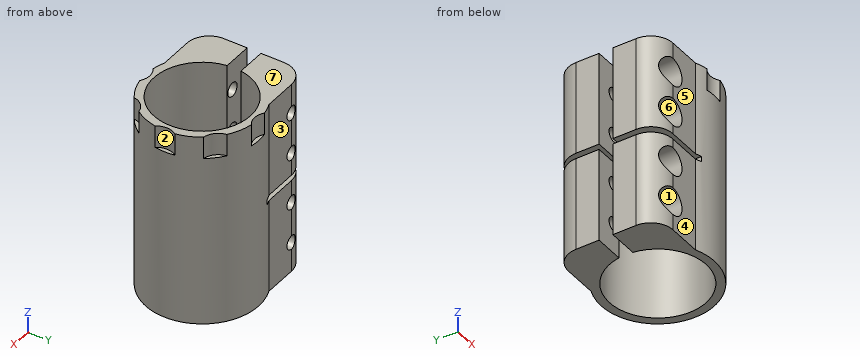
from build123d import *

# Parameters (mm, degrees)
F1_DEPTH       = 35
F3_D           = 5
F3_START       = 1.8205079
F3_CBORE_D     = 10
F3_CBORE_DEPTH = 8
F4_W           = 22.4
F4_H           = 2
F5_DEPTH       = 25
F6_R           = 6
F7_DEPTH       = 8


with BuildPart() as f1:
    # F0 (on Top) → F1 (new body, symmetric)
    with BuildSketch(Plane.XY):
        with BuildLine():
            Line((-20.1192642082, -18.9086026559), (-7.9192642082, -18.9086026559))
            ThreePointArc((-7.9192642082, -18.9086026559), (20.5, 0), (-7.9192642082, 18.9086026559))
            Line((-7.9192642082, 18.9086026559), (-20.1192642082, 18.9086026559))
            ThreePointArc((-20.1192642082, 18.9086026559), (-25.7761184577, 16.5654569054), (-28.1192642082, 10.9086026559))
            Line((-28.1192642082, 10.9086026559), (-28.1192642082, 2.5086026559))
            Line((-28.1192642082, 2.5086026559), (-17.3192642082, 2.5086026559))
            ThreePointArc((-17.3192642082, 2.5086026559), (17.5, 0), (-17.3192642082, -2.5086026559))
            Line((-17.3192642082, -2.5086026559), (-28.1192642082, -2.5086026559))
            Line((-28.1192642082, -2.5086026559), (-28.1192642082, -10.9086026559))
            ThreePointArc((-28.1192642082, -10.9086026559), (-25.7761184577, -16.5654569054), (-20.1192642082, -18.9086026559))
        make_face()
    extrude(amount=F1_DEPTH, both=True)

    # F3 (through all)
    # its depths count from where the whole tool has entered the part; down to there all is cleared
    with Locations(Plane.XZ.offset(18.9086026559).offset(-F3_START)):
        with Locations((-20.2, -24.25), (-20.2, -9.25), (-20.2, 9.25), (-20.2, 24.25)):
            CounterBoreHole(F3_D / 2, F3_CBORE_D / 2, F3_CBORE_DEPTH)

    # F4 (on Front) → F5 (cut, symmetric)
    with BuildSketch(Plane.XZ):
        with Locations((-16.9192642082, 0)):
            Rectangle(F4_W, F4_H)
    extrude(amount=F5_DEPTH, both=True, mode=Mode.SUBTRACT)

    # F6 (on face) → F7 (cut)
    with BuildSketch(Plane.XY.offset(35)):
        with Locations((0, -25)):
            Circle(F6_R)
        with Locations((17.6776695297, -17.6776695297)):
            Circle(F6_R)
        with Locations((25, 0)):
            Circle(F6_R)
        with Locations((17.6776695297, 17.6776695297)):
            Circle(F6_R)
        with Locations((0, 25)):
            Circle(F6_R)
    extrude(amount=-F7_DEPTH, mode=Mode.SUBTRACT)


solid = f1.part
Verification items for the finished model (mm, model axes). Face numbers are marked on the shaded views. A direction names the side the tool comes from. Coordinates: 2 decimals unless noted, no trailing zeros. Write each loop counter-clockwise with the first axis right and the second up, starting at its lowest first coordinate (ties: lowest second). Pieces come first, ordered by that corner, then holes. Notation, with made-up numbers: (11.5, -37) -> (51.5, -37) arc R26 ccw to (51.5, -18) -> close; hole circle Ø3 at (61.25, 39). An arc over 180 degrees is marked (long way). One line per item, written item: value. Start each with the question number.
Q1. Mould release check, pull along Z, two halves, no side actions. Record for the marked faces 5, 6 and 7: pulls with the +Z half, pulls with the -Z half, needs draft (parallel to the pull), parting line crosses it, or undercut.
Q2. Cross-section at D-D on z = 25.5. Enter the section's corners in (x, y).
Q3. Cross-section at C-C on x = 8.5. Enter the section's corners in (y, z), and give its area (3 significant figures).
Q4. Thickness scan on L1, parallel to Z at x = -20.2, y = -16.75; L2, parallel to Z at x = -20, y = -5; L3, parallel to X at y = 14.75, z = -9.25. Record the ranges inside material, lowest first. Write a range as from..to.
Q5. Cross-section at B-B on z = -16. Enter the section's corners in (x, y).
Q6. Go/stop test with flat-tipped pins: P1, Ø3, axis at x = 4, z = 12, coming from the +Y side; P2, Ø5.5, axis at x = -20.5, z = -15, coming from the +Y side; P3, Ø1.6, axis at y = 19, z = 0, coming from the -X side. Record where each tip stops, or that it passes through.
Q7. Access from +Z, -Z, +X, -X, +Y, -Y to the whole of each face (thin tool, end or side, straight path). Record for the marked faces 1, 2, 3 and 4.
Q8. Cross-section at A-A on y = 14. Enter the section's corners in (x, z).
Checked values:
1. face 5: needs draft
1. face 6: undercut
1. face 7: pulls with the +Z half
2. outline: (-28.12, -10.91) arc R8 ccw to (-25.04, -17.22) -> (-25.04, -9.09) -> (-22.37, -9.09) -> (-22.37, -2.51) -> (-28.12, -2.51) -> close; (-28.12, 2.51) -> (-22.37, 2.51) -> (-22.37, 18.59) arc R8 ccw to (-28.12, 10.91) -> close; (-18.03, -9.09) -> (-15.36, -9.09) -> (-15.36, -18.91) -> (-7.92, -18.91) arc R20.5 ccw (long way) to (-7.92, 18.91) -> (-18.03, 18.91) -> (-18.03, 2.51) -> (-17.32, 2.51) arc R17.5 cw (long way) to (-17.32, -2.51) -> (-18.03, -2.51) -> close
3. outline: (-18.65, -35) -> (-15.3, -35) -> (-15.3, 35) -> (-18.65, 35) -> close; (15.3, -35) -> (18.65, -35) -> (18.65, 35) -> (15.3, 35) -> close
3. area: 470 mm²
4. L1: z = -35..-29.25, -19.25..-14.25, -4.25..-1, 1..4.25, 14.25..19.25, 29.25..35
4. L2: z = -35..-26.74, -21.76..-11.74, -6.76..-1, 1..6.76, 11.74..21.76, 26.74..35
4. L3: x = -27.14..-22.7, -17.7..-9.42, 9.42..14.24
5. outline: (-28.12, -10.91) arc R8 ccw to (-20.12, -18.91) -> (-7.92, -18.91) arc R20.5 ccw (long way) to (-7.92, 18.91) -> (-20.12, 18.91) arc R8 ccw to (-28.12, 10.91) -> (-28.12, 2.51) -> (-17.32, 2.51) arc R17.5 cw (long way) to (-17.32, -2.51) -> (-28.12, -2.51) -> close
6. P1: stops at y = 20.35
6. P2: stops at y = 18.91
6. P3: stops at x = -5.72
7. face 1: -Y
7. face 2: +Z, +X
7. face 3: +Z, -Z, -X, +Y
7. face 4: +Z, -Z, -X, -Y
8. outline: (-27.5, -35) -> (-10.5, -35) -> (-10.5, -1) -> (-27.5, -1) -> close; (-27.5, 1) -> (-10.5, 1) -> (-10.5, 35) -> (-27.5, 35) -> close; (10.5, -35) -> (14.97, -35) -> (14.97, 27) -> (12.94, 27) -> (12.94, 35) -> (10.5, 35) -> close; hole circle Ø5 at (-20.2, -24.25); hole circle Ø5 at (-20.2, -9.25); hole circle Ø5 at (-20.2, 9.25); hole circle Ø5 at (-20.2, 24.25)
